Print and shaded views of the part. All mm, measured from the part's lowest x, y and z. Give positions to 0.01 mm unless a question says otherwise; leave off trailing zeros. Loops run counter-clockwise (first coordinate to the right, second up) from the corner with the lowest first, then second, coordinate; pieces in that order, holes last. Notation, with made-up numbers: M -18.75,77 L 16.25,77 A34 ccw 16.25,116 Z; hole C 15.5,47.5 d7. An arc over 180 degrees is marked long. Put each result on its own line as item: value. Start each with the question number.
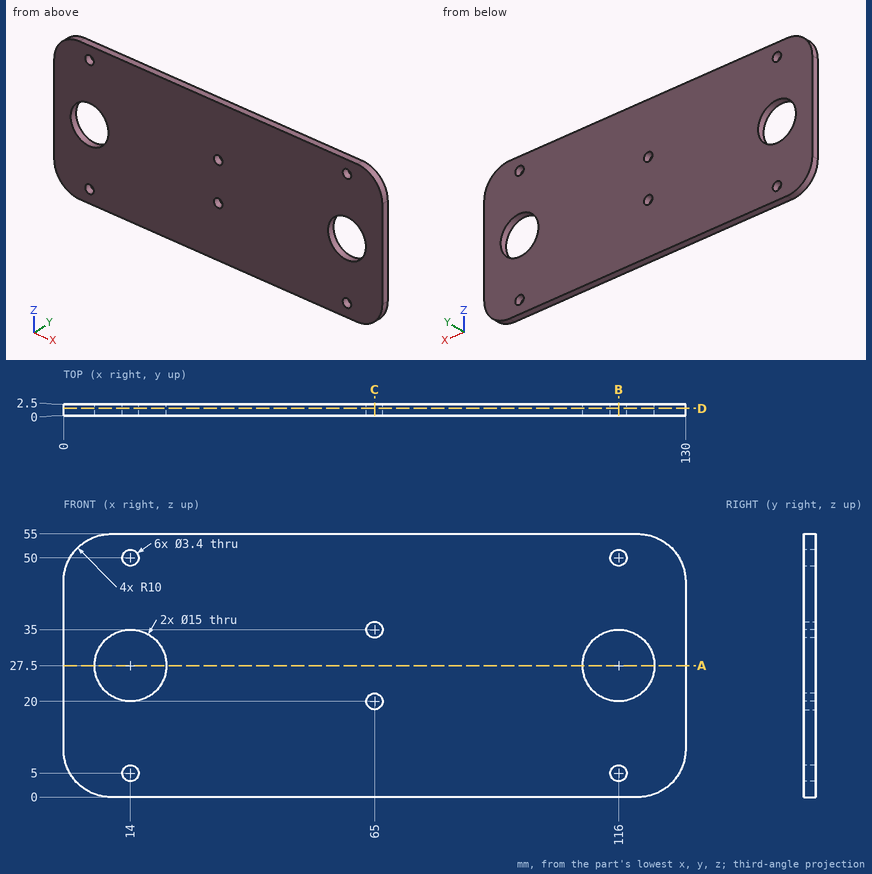
1) Band-saw the part on B-B on x = 116. Give the cut face in (y, z).
2) Pin check, flat tips, straight feed: pin 1 Ø2.5 at (x, z) = (116, 5) entering from -Y; pin 2 Ø4.5 at (x, z) = (14, 5) entering from -Y. Stop position of each tip, or through.
3) Band-saw the part on D-D on y = 1.6. State how many separate pieces and enclosed holes the cut face has, then the cut area to 3 significant figures.
4) Band-saw the part on A-A on z = 27.5. Give the cut face in (x, y), then the cut area to 3 significant figures.
5) Band-saw the part on C-C on x = 65. Give the cut face in (y, z), then the cut area to 4 significant figures.
6) Wall check: L1, parallel to Z at x = 116, y = 1.9; L2, parallel to Z at x = 65, y = 1.2; L3, parallel to X at y = 0.5, z = 22. Give the ranges that are in metal, low to high.
Evaluation:
1. outline: M 0,0 L 2.5,0 L 2.5,3.3 L 0,3.3 Z; M 0,6.7 L 2.5,6.7 L 2.5,20 L 0,20 Z; M 0,35 L 2.5,35 L 2.5,48.3 L 0,48.3 Z; M 0,51.7 L 2.5,51.7 L 2.5,55 L 0,55 Z
2. pin 1: through
2. pin 2: y = 0
3. separate pieces: 1
3. enclosed holes: 8
3. area: 6,660 mm2
4. outline: M 0,0 L 6.5,0 L 6.5,2.5 L 0,2.5 Z; M 21.5,0 L 108.5,0 L 108.5,2.5 L 21.5,2.5 Z; M 123.5,0 L 130,0 L 130,2.5 L 123.5,2.5 Z
4. area: 250 mm2
5. outline: M 0,0 L 2.5,0 L 2.5,18.3 L 0,18.3 Z; M 0,21.7 L 2.5,21.7 L 2.5,33.3 L 0,33.3 Z; M 0,36.7 L 2.5,36.7 L 2.5,55 L 0,55 Z
5. area: 120.5 mm2
6. L1: 0 to 3.3, 6.7 to 20, 35 to 48.3, 51.7 to 55
6. L2: 0 to 18.3, 21.7 to 33.3, 36.7 to 55
6. L3: 0 to 8.9, 19.1 to 110.9, 121.1 to 130
